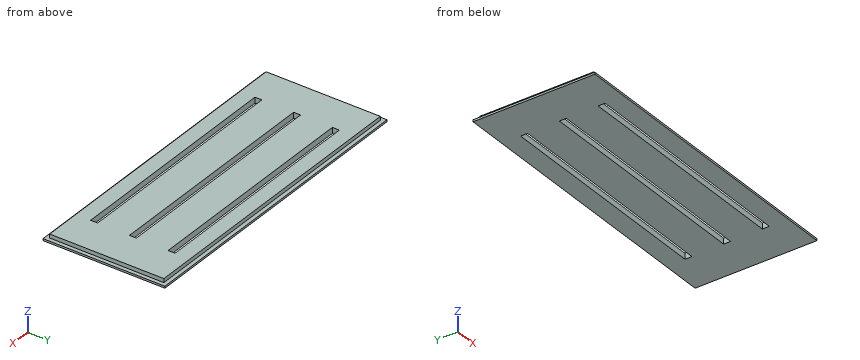
from build123d import *

# Parameters (mm, degrees)
F0_W     = 79.5
F0_H     = 31.5
F0_W_2   = 77.5
F0_H_2   = 29.5
F0_W_3   = 58.807618
F0_H_3   = 1.786274
F1_DEPTH = 0.5
F2_DEPTH = 1


with BuildPart() as f1:
    # F0 (on Top) → F1 (new body)
    with BuildSketch(Plane.XY):
        Rectangle(F0_W, F0_H)
        Rectangle(F0_W_2, F0_H_2, mode=Mode.SUBTRACT)
        Rectangle(F0_W_2, F0_H_2)
        with Locations((0, -10)):
            Rectangle(F0_W_3, F0_H_3, mode=Mode.SUBTRACT)
        Rectangle(F0_W_3, F0_H_3, mode=Mode.SUBTRACT)
        with Locations((0, 10)):
            Rectangle(F0_W_3, F0_H_3, mode=Mode.SUBTRACT)
    extrude(amount=-F1_DEPTH)

    # F0 (on Top) → F2 (join)
    with BuildSketch(Plane.XY):
        Rectangle(F0_W_2, F0_H_2)
        with Locations((0, -10)):
            Rectangle(F0_W_3, F0_H_3, mode=Mode.SUBTRACT)
        Rectangle(F0_W_3, F0_H_3, mode=Mode.SUBTRACT)
        with Locations((0, 10)):
            Rectangle(F0_W_3, F0_H_3, mode=Mode.SUBTRACT)
    extrude(amount=F2_DEPTH)


solid = f1.part
Can you work these out from the model? Positions are in its coordinate system, mm. Round coordinates to 2 decimals unless told otherwise and drop trailing zeros. Order: outer loops, then holes, each group sorted by start corner. A loop starts at its lowest first (then second) coordinate and runs counter-clockwise, first axis right, second up. Notation, with made-up numbers: (-29, -16.5) - (4, -16.5) arc R23 ccw to (4, 22.5) - close; hole circle Ø4 at (-3.5, 67). An arc over 180 degrees is marked (long way). Answer in a Markdown table with one row per item.
(1) Suppose I cut it at C-C, the plane x = -34.5. Please give me the cut outline in (y, z).
From the geometry:
| item | result |
|---|---|
| outline | (-15.75, -0.5) - (15.75, -0.5) - (15.75, 0) - (14.75, 0) - (14.75, 1) - (-14.75, 1) - (-14.75, 0) - (-15.75, 0) - close |
(2) Suppose I cut it at A-A, the plane z = 0.7. Please give me the cut outline in (x, y), plus the area to 3 significant figures.
From the geometry:
| item | result |
|---|---|
| outline | (-38.75, -14.75) - (38.75, -14.75) - (38.75, 14.75) - (-38.75, 14.75) - close; hole (-29.4, -10.89) - (29.4, -10.89) - (29.4, -9.11) - (-29.4, -9.11) - close; hole (-29.4, -0.89) - (29.4, -0.89) - (29.4, 0.89) - (-29.4, 0.89) - close; hole (-29.4, 9.11) - (29.4, 9.11) - (29.4, 10.89) - (-29.4, 10.89) - close |
| area | 1,970 mm2 |
(3) Suppose I cut it at D-D, the plane y = 13.5. Please give me the cut outline in (x, z).
From the geometry:
| item | result |
|---|---|
| outline | (-39.75, -0.5) - (39.75, -0.5) - (39.75, 0) - (38.75, 0) - (38.75, 1) - (-38.75, 1) - (-38.75, 0) - (-39.75, 0) - close |
(4) For P1, Ø0.5, axis at y = -6, z = 0.5, coming from the -X side; P2, Ø0.5, axis at x = 9.5, z = 0.5, coming from the -Y side, each with a flat end and sliding along its axis, tell me the tip position at first contact or that it passes through.
From the geometry:
| item | result |
|---|---|
| P1 | stops at x = -38.75 |
| P2 | stops at y = -14.75 |
(5) Please list where these lines run through material, in increasing order: L1, parallel to Y at x = 15, z = 0.25; L2, parallel to Y at x = -11.5, z = -0.1; L3, parallel to X at y = -2, z = 0.9. Write a range as from..to.
From the geometry:
| item | result |
|---|---|
| L1 | y = -14.75..-10.89, -9.11..-0.89, 0.89..9.11, 10.89..14.75 |
| L2 | y = -15.75..-10.89, -9.11..-0.89, 0.89..9.11, 10.89..15.75 |
| L3 | x = -38.75..38.75 |
(6) Suppose I cut it at B-B, the plane x = -22. Please give me the cut outline in (y, z).
From the geometry:
| item | result |
|---|---|
| outline | (-15.75, -0.5) - (-10.89, -0.5) - (-10.89, 1) - (-14.75, 1) - (-14.75, 0) - (-15.75, 0) - close; (-9.11, -0.5) - (-0.89, -0.5) - (-0.89, 1) - (-9.11, 1) - close; (0.89, -0.5) - (9.11, -0.5) - (9.11, 1) - (0.89, 1) - close; (10.89, -0.5) - (15.75, -0.5) - (15.75, 0) - (14.75, 0) - (14.75, 1) - (10.89, 1) - close |
